Autodesk Inventor part; units mm, degrees
ref_plane "YZ Plane" through (0, 0, 0) normal (1, 0, 0) x (0, 1, 0)
ref_plane "XZ Plane" through (0, 0, 0) normal (0, 1, 0) x (-1, 0, 0)
ref_plane "XY Plane" through (0, 0, 0) normal (0, 0, 1) x (1, 0, 0)
sketch "Schizzo2" plane through (0, 0, 0) normal (0, 0, 1) x (1, 0, 0)
  line L0 (0, 0) -> (0, 1.5)
  line L1 (0, 1.5) -> (1.5667, 1.5)
  line L2 (0, 0) -> (2.35, 0)
  arc A0 (2.35, 0) -> (1.5667, 1.5) centre (0.5222, 0) ccw
  dimension "d0" = 2.35
  dimension "d1" = 1.5
  dimension "d2" = 1.5667
revolve "Rivoluzione1" add sketch "Schizzo2" angle 360 about axis through (0, 0, 0) along (0, 1, 0)
sketch "Schizzo3" plane through (0, 0, 0) normal (0, -1, 0) x (1, 0, 0)
  circle A0 centre (0, 0) radius 1.5667
  circle A1 centre (0, 0) radius 1.25
  dimension "d4" = 2.5
extrude "Estrusione1" add sketch "Schizzo3" along normal blind 4 contours A1
thread "Filettatura1"
chamfer "Smusso1" distance 0.25 angle 45 1 edges at (-1.25, -4, 0) measured on face at (-0.1478, -4, -0.3896)
sketch "Schizzo4" plane through (0, 1.5, 0) normal (0, 1, 0) x (1, 0, 0)
  circle A0 centre (0, 0) radius 1.25
  line L0 (0.4503, 0.78) -> (0.9007, 0)
  line L1 (0.9007, 0) -> (0.4503, -0.78)
  line L2 (0.4503, -0.78) -> (-0.4503, -0.78)
  line L3 (-0.4503, -0.78) -> (-0.9007, 0)
  line L4 (-0.9007, 0) -> (-0.4503, 0.78)
  line L5 (-0.4503, 0.78) -> (0.4503, 0.78)
  dimension "d12" = 1.56
extrude "Estrusione2" cut sketch "Schizzo4" against normal blind 0.8 contours L0 L1 L2 L3 L4 L5
equation "\"d0\" = 0.5 * dk"
equation "\"d1\" = k"
equation "\"d2\" = 0.333333 * dk"
equation "\"d4\" = d"
equation "\"d5\" = L"
equation "\"d12\" = es"
equation "\"d13\" = t"
equation "\"t\" = 0.8"
equation "\"k\" = 1.5"
equation "\"d\" = 2.5"
equation "\"dk\" = 4.7"
equation "\"es\" = 1.56"
equation "\"L\" = 4"
properties part number "Vite ISO 7380"
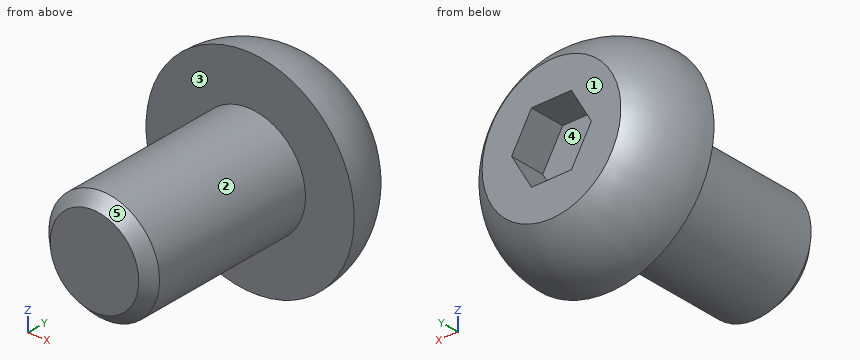
Here's how the part is built. I have some questions about the finished solid (model axes, mm). Face numbers are marked on the shaded views. A direction names the side the tool comes from. Round coordinates to 2 decimals unless told otherwise and drop trailing zeros. Loops run counter-clockwise (first coordinate to the right, second up) from the corner with the lowest first, then second, coordinate; pieces in that order, holes last.
1. Suppose I cut it at A-A, the plane y = -1.75. Please give me the cut outline in (x, z), and give its area (3 significant figures).
Answers:
outline: circle Ø2.5 at (0, 0)
area: 4.91 mm2
2. Thinking about a two-plate mould opening in Z: for the marked faces 3, 4 and 5, which applies, released by +Z, released by -Z, zero draft, split by the parting line, or undercut?
Answers:
face 3: zero draft
face 4: undercut
face 5: split by the parting line
3. For the marked faces 1 and 2, which set-ups out of +Z, -Z, +X, -X, +Y, -Y let a thin tool reach every point of the face, with its end or its side?
Answers:
face 1: +Z, -Z, +X, -X, +Y
face 2: -Y
4. If I drill on probe 1 along X at (y, z) = (-1.2, -0.05); probe 2 along Y at (x, z) = (-1.4, 0.6); probe 3 along Y at (x, z) = (-0.9, -1.7), over which ranges is the centre line in solid material (lowest first)?
Answers:
probe 1: x = -1.25 to 1.25
probe 2: y = 0 to 1.5
probe 3: y = 0 to 1.17
5. Will these pins go through, and if not, where does the flat tip stop? pin 1 (1.5 mm diameter, centred on x = -1.5, z = -1.5, fed in from -Y); pin 2 (2 mm diameter, centred on x = -1.5, y = -2.5, fed in from +Z); pin 3 (0.9 mm diameter, centred on x = 0, y = 1, fed in from -Z).
Answers:
pin 1: stops at y = 0
pin 2: stops at z = 1.15
pin 3: stops at z = -2.27
